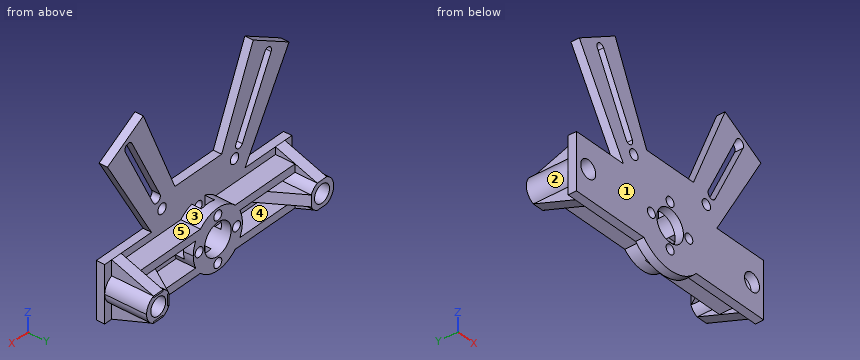
from build123d import *

# Parameters (mm, degrees)
SKETCH_1_R          = 3.2
SKETCH_1_R_2        = 1.8
SKETCH_1_R_3        = 5.7
SKETCH_1_R_4        = 1.7
EXTRUDE_1_DEPTH     = 3
SKETCH_2_R          = 10.5
EXTRUDE_2_DEPTH     = 7
SKETCH_4_R          = 1.7
CUT_EXTRUDE_1_DEPTH = 7
CUT_EXTRUDE_2_DEPTH = 3.5
SKETCH_6_R          = 5.7
CUT_EXTRUDE_3_DEPTH = 20
SKETCH_7_R          = 5
SKETCH_7_R_2        = 3.2
EXTRUDE_3_DEPTH     = 15
SKETCH_8_W          = 10
SKETCH_8_H          = 4
SKETCH_8_W_2        = 4
SKETCH_8_H_2        = 6
EXTRUDE_4_DEPTH     = 15
CUT_EXTRUDE_4_DEPTH = 15
CUT_EXTRUDE_5_DEPTH = 15
CUT_EXTRUDE_6_DEPTH = 15
SKETCH_12_W         = 25.575378798
SKETCH_12_H         = 2.842045507
EXTRUDE_5_DEPTH     = 7


with BuildPart() as part:
    # 草图1 → 凸台-拉伸1 (new body)
    with BuildSketch(Plane(origin=(0, 0, 0), x_dir=(1, 0, 0), z_dir=(0, 1, 0))):
        with BuildLine():
            Line((-35.081832586, -10), (-40, -10))
            Line((-40, -10), (-40, 10))
            Line((-40, 10), (-11.180339887, 10))
            ThreePointArc((-11.180339887, 10), (0, 15), (11.180339887, 10))
            Line((11.180339887, 10), (40, 10))
            Line((40, 10), (40, -10))
            Line((40, -10), (20, -10))
            Line((20, -10), (38.795982487, -42.134997854))
            Line((38.795982487, -42.134997854), (23.493176713, -51.085714784))
            Line((23.493176713, -51.085714784), (10.00055485, -20.000324527))
            Line((10.00055485, -20.000324527), (-9.99944515, -20.000324527))
            Line((-9.99944515, -20.000324527), (-23.493239928, -51.085714784))
            Line((-23.493239928, -51.085714784), (-38.79573581, -42.1354119))
            Line((-38.79573581, -42.1354119), (-20, -10))
            Line((-20, -10), (-35.081832586, -10))
        make_face()
        with Locations((35, 0)):
            Circle(SKETCH_1_R, mode=Mode.SUBTRACT)
        with Locations((-15.5, -15.5)):
            Circle(SKETCH_1_R_2, mode=Mode.SUBTRACT)
        with Locations((15.5, -15.5)):
            Circle(SKETCH_1_R_2, mode=Mode.SUBTRACT)
        with Locations((-35, 0)):
            Circle(SKETCH_1_R, mode=Mode.SUBTRACT)
        Circle(SKETCH_1_R_3, mode=Mode.SUBTRACT)
        with Locations((-8, 0)):
            Circle(SKETCH_1_R_4, mode=Mode.SUBTRACT)
        with Locations((0, 8)):
            Circle(SKETCH_1_R_4, mode=Mode.SUBTRACT)
        with Locations((8, 0)):
            Circle(SKETCH_1_R_4, mode=Mode.SUBTRACT)
        with Locations((0, -8)):
            Circle(SKETCH_1_R_4, mode=Mode.SUBTRACT)
        with BuildLine():
            Line((-16.131862345, -20.121977189), (-28.419219954, -44.445930008))
            ThreePointArc((-28.419219954, -44.445930008), (-30.461319047, -45.117305053), (-31.132694091, -43.07520596))
            Line((-31.132694091, -43.07520596), (-18.845336482, -18.75125314))
            ThreePointArc((-18.845336482, -18.75125314), (-16.803237389, -18.079878096), (-16.131862345, -20.121977189))
        make_face(mode=Mode.SUBTRACT)
        with BuildLine():
            Line((19.251434516, -19.436615165), (31.203359651, -43.037711333))
            ThreePointArc((31.203359651, -43.037711333), (30.498813674, -45.187970612), (28.348554395, -44.483424635))
            Line((28.348554395, -44.483424635), (16.39662926, -20.882328467))
            ThreePointArc((16.39662926, -20.882328467), (17.101175237, -18.732069188), (19.251434516, -19.436615165))
        make_face(mode=Mode.SUBTRACT)
    extrude(amount=EXTRUDE_1_DEPTH)

    # 草图2 → 凸台-拉伸2 (add)
    with BuildSketch(Plane(origin=(0, 3, 0), x_dir=(1, 0, 0), z_dir=(0, 1, 0))):
        Circle(SKETCH_2_R)
    extrude(amount=EXTRUDE_2_DEPTH)

    # 草图4 → 切除-拉伸1 (cut)
    with BuildSketch(Plane.XZ.offset(-3)):
        with Locations((0, -8)):
            Circle(SKETCH_4_R)
        with Locations((-8, 0)):
            Circle(SKETCH_4_R)
        with Locations((8, 0)):
            Circle(SKETCH_4_R)
        with Locations((0, 8)):
            Circle(SKETCH_4_R)
    extrude(amount=-CUT_EXTRUDE_1_DEPTH, mode=Mode.SUBTRACT)

    # 草图5 → 切除-拉伸2 (cut)
    with BuildSketch(Plane(origin=(0, 3, 0), x_dir=(1, 0, 0), z_dir=(0, 1, 0))):
        Polygon((-4.766838493, 0), (-6.383419246, 2.8), (-11.233161507, 2.8), (-11.233161507, -2.8), (-6.383419246, -2.8), align=None)
        Polygon((4.766838493, 0), (6.383419246, -2.8), (11.233161507, -2.8), (11.233161507, 2.8), (6.383419246, 2.8), align=None)
        Polygon((-2.8, 11.233161507), (-2.8, 6.383419246), (0, 4.766838493), (2.8, 6.383419246), (2.8, 11.233161507), align=None)
        Polygon((0, -4.766838493), (-2.8, -6.383419246), (-2.8, -11.233161507), (2.8, -11.233161507), (2.8, -6.383419246), align=None)
    extrude(amount=CUT_EXTRUDE_2_DEPTH, mode=Mode.SUBTRACT)

    # 草图6 → 切除-拉伸3 (cut)
    with BuildSketch(Plane.XZ.offset(-3)):
        Circle(SKETCH_6_R)
    extrude(amount=-CUT_EXTRUDE_3_DEPTH, mode=Mode.SUBTRACT)

    # 草图7 → 凸台-拉伸3 (add)
    with BuildSketch(Plane(origin=(0, 3, 0), x_dir=(1, 0, 0), z_dir=(0, 1, 0))):
        with Locations((-35, 0)):
            Circle(SKETCH_7_R)
        with Locations((-35, 0)):
            Circle(SKETCH_7_R_2, mode=Mode.SUBTRACT)
        with Locations((35, 0)):
            Circle(SKETCH_7_R)
        with Locations((35, 0)):
            Circle(SKETCH_7_R_2, mode=Mode.SUBTRACT)
    extrude(amount=EXTRUDE_3_DEPTH)

    # 草图8 → 凸台-拉伸4 (add)
    with BuildSketch(Plane(origin=(0, 3, 0), x_dir=(1, 0, 0), z_dir=(0, 1, 0))):
        with Locations((-26, 0)):
            Rectangle(SKETCH_8_W, SKETCH_8_H)
        with Locations((-35, 7)):
            Rectangle(SKETCH_8_W_2, SKETCH_8_H_2)
        with Locations((-35, -7)):
            Rectangle(SKETCH_8_W_2, SKETCH_8_H_2)
        with Locations((26, 0)):
            Rectangle(SKETCH_8_W, SKETCH_8_H)
        with Locations((35, 7)):
            Rectangle(SKETCH_8_W_2, SKETCH_8_H_2)
        with Locations((35, -7)):
            Rectangle(SKETCH_8_W_2, SKETCH_8_H_2)
    extrude(amount=EXTRUDE_4_DEPTH)

    # 草图9 → 切除-拉伸4 (cut)
    with BuildSketch(Plane.XY.offset(2)):
        Polygon((-30.417424305, 18), (-21, 3), (-21, 18), align=None)
        Polygon((21, 3), (30.417424305, 18), (21, 18), align=None)
    extrude(amount=-CUT_EXTRUDE_4_DEPTH, mode=Mode.SUBTRACT)

    # 草图10 → 切除-拉伸5 (cut)
    with BuildSketch(Plane.ZY.offset(-33)):
        Polygon((-4.582575695, 18), (-10, 3), (-10, 18), align=None)
        Polygon((4.582575695, 18), (10, 18), (10, 3), align=None)
    extrude(amount=-CUT_EXTRUDE_5_DEPTH, mode=Mode.SUBTRACT)

    # 草图11 → 切除-拉伸6 (cut)
    with BuildSketch(Plane(origin=(-33, 0, 0), x_dir=(0, 0, -1), z_dir=(1, 0, 0))):
        Polygon((-4.582575695, 18), (-10, 3), (-10, 18), align=None)
        Polygon((4.582575695, 18), (10, 3), (10, 18), align=None)
    extrude(amount=-CUT_EXTRUDE_6_DEPTH, mode=Mode.SUBTRACT)

    # 草图12 → 凸台-拉伸5 (add)
    with BuildSketch(Plane(origin=(0, 3, 0), x_dir=(1, 0, 0), z_dir=(0, 1, 0))):
        with Locations((-20.212310601, -6.003598449)):
            Rectangle(SKETCH_12_W, SKETCH_12_H)
        with Locations((-20.212310601, 6.003598449)):
            Rectangle(SKETCH_12_W, SKETCH_12_H)
        with Locations((20.212310601, 6.003598449)):
            Rectangle(SKETCH_12_W, SKETCH_12_H)
        with Locations((20.212310601, -6.003598449)):
            Rectangle(SKETCH_12_W, SKETCH_12_H)
    extrude(amount=EXTRUDE_5_DEPTH)


solid = part.part
Check sheet for the modelled part. Datum: model origin and axes. Units: mm. Face numbers are marked on the shaded views. A direction names the side the tool comes from. Give positions to 0.01 mm unless a question says otherwise; leave off trailing zeros. Write each loop counter-clockwise with the first axis right and the second up, starting at its lowest first coordinate (ties: lowest second). Pieces come first, ordered by that corner, then holes. Notation, with made-up numbers: (74, 39) -> (85, 39) arc R28 cw to (85, 67) -> close; hole circle Ø8 at (42, 33). An arc over 180 degrees is marked (long way). One line per item, written item: value. Start each with the question number.
Item 1: Tool access check on the marked faces 4 and 5. Record the directions out of +Z, -Z, +X, -X, +Y, -Y that give a thin tool (end or side, any length) a straight path to the whole face; none if there is none.
Item 2: Material ranges on probe 1 along Z at (x, y) = (0, 7.2); probe 2 along Z at (x, y) = (0, 1.1); probe 3 along Y at (x, z) = (-8.5, -2.5), recorded low to high. Write a range as from..to.
Item 3: Section check C-C on z = 15.5. Record the cut outline in (x, y).
Item 4: Gauge pin test, flat ends, axial feed: pin 1 (3.5 mm diameter, centred on x = 18, y = 6.5, fed in from +Z); pin 2 (3 mm diameter, centred on y = 4, z = -8.5, fed in from -X); pin 3 (6 mm diameter, centred on y = 3, z = 16.5, fed in from -X); pin 4 (8 mm diameter, centred on y = 4.5, z = 20, fed in from +X). Record the tip position at first contact, or that the pin passes through.
Item 5: Section check B-B on x = 35. Record the cut outline in (y, z).
Item 6: Draft check along X on the marked faces 1, 2 and 3. Enter one of: +X half, -X half, draft (parallel to the pull), parting line (faces both ways), or undercut.
Item 7: Section check A-A on x = 0. State how many separate pieces and enclosed holes the cut face has, then the cut area to 3 significant figures.
Results list:
1. face 4: +Y
1. face 5: +Z, +Y
2. probe 1: -10.5..-9.7, -6.3..-5.7, 5.7..6.3, 9.7..10.5
2. probe 2: -15..-9.7, -6.3..-5.7, 5.7..6.3, 9.7..20
2. probe 3: 0..3, 6.5..10
3. outline: (-23.22, 0) -> (-17.3, 0) -> (-17.3, 3) -> (-23.22, 3) -> close; (-13.7, 0) -> (13.7, 0) -> (13.7, 3) -> (-13.7, 3) -> close; (17.3, 0) -> (23.22, 0) -> (23.22, 3) -> (17.3, 3) -> close
4. pin 1: z = 7.42
4. pin 2: x = -40
4. pin 3: x = -25.56
4. pin 4: x = 28.02
5. outline: (0, -10) -> (3, -10) -> (18, -4.58) -> (18, -3.2) -> (0, -3.2) -> close; (0, 3.2) -> (18, 3.2) -> (18, 4.58) -> (3, 10) -> (0, 10) -> close; (0, 35.65) -> (3, 35.65) -> (3, 44.36) -> (0, 44.36) -> close
6. face 1: draft
6. face 2: -X half
6. face 3: undercut
7. separate pieces: 8
7. enclosed holes: 0
7. area: 60.2 mm²
